The model under review builds one solid part; all positions refer to its coordinate system, in mm. A direction names the side the tool comes from. Round coordinates to 2 decimals unless told otherwise and drop trailing zeros. Loops run counter-clockwise (first coordinate to the right, second up) from the corner with the lowest first, then second, coordinate; pieces in that order, holes last. Notation, with made-up numbers: (77, 31.25) -> (136, 31.25) arc R18 cw to (136, 41.25) -> close; hole circle Ø3 at (73.25, 67). An arc over 180 degrees is marked (long way). Use a Markdown table: item, result. Add a question column.
1) Consider section D-D on y = 2.45. State how many separate pieces and enclosed holes the cut face has, plus the area to 3 significant figures.
2) For faces 1 (the flat face through (25, 1, 24)), 2 (the flat face through (9.833, 1, -23)), 3 (the flat face through (26.5, 1, 0)), list the 3-axis set-ups (+Z, -Z, +X, -X, +Y, -Y) from which the entire face can be reached by the end or side of a thin tool; tool diameter is ignored.
3) Wall thickness on probe 1 along X at (y, z) = (1.3, -15.69); probe 2 along Z at (x, y) = (-8, 0.5); probe 3 along X at (y, z) = (2.8, -22.5): over which ranges is each line inside the solid? List them lowest first.
4) Mouldability with a two-part tool opening along Z and no side actions: class faces 4 (the flat face through (29.5, 1, 16)), 5 (the flat face through (-26.5, 1, 0)), 6 (the flat face through (-28, 1, -8)), 7 (the flat face through (0, 2, -33)) as released by +Z, released by -Z, zero draft, split by the parting line, or undercut.
5) Insertion check: pin 1 (1.5 mm diameter, centred on x = -21, y = 0.5, fed in from -Z); pin 2 (0.9 mm diameter, centred on x = 26, y = 1, fed in from +Z); pin 3 (1.5 mm diameter, centred on y = 1.5, z = 1, fed in from +X). Each pin has a flat end and moves straight along its axis. Give the tip position at first contact, or say it passes through.
6) Consider section B-B on x = 0. Give the boundary of the cut face in (y, z).
7) Consider section C-C on z = -15.69. Give the boundary of the cut face in (x, y).
8) Consider section A-A on z = 28.5. Give the boundary of the cut face in (x, y).
from build123d import *

# Parameters (mm, degrees)
SKETCH1_R           = 1.6
BOSS_EXTRUDE1_DEPTH = 3
SKETCH2_R           = 2.1
BOSS_EXTRUDE2_DEPTH = 3


with BuildPart() as part:
    # Sketch1 → Boss-Extrude1 (new body)
    with BuildSketch(Plane(origin=(0, 0, 0), x_dir=(1, 0, 0), z_dir=(0, 1, 0))):
        Polygon((-29.5, 24), (-29.5, 8), (-26.5, 8), (-26.5, -8), (-29.5, -8), (-29.5, -24), (-9.833333333, -24), (-9.833333333, -21), (9.833333333, -21), (9.833333333, -24), (29.5, -24), (29.5, -8), (26.5, -8), (26.5, 8), (29.5, 8), (29.5, 24), (9.833333333, 24), (9.833333333, 21), (-9.833333333, 21), (-9.833333333, 24), align=None)
        with Locations(Location((-21.0185, 15.69, 0), (0, 0, 270))):
            Circle(SKETCH1_R, mode=Mode.SUBTRACT)
        with Locations(Location((21.0185, 15.69, 0), (0, 0, 270))):
            Circle(SKETCH1_R, mode=Mode.SUBTRACT)
        with Locations(Location((21.0185, -13.52, 0), (0, 0, 270))):
            Circle(SKETCH1_R, mode=Mode.SUBTRACT)
    extrude(amount=BOSS_EXTRUDE1_DEPTH)

    # Sketch2 → Boss-Extrude2 (add)
    with BuildSketch(Plane(origin=(0, 3, 0), x_dir=(1, 0, 0), z_dir=(0, 1, 0))):
        Polygon((-19.666666667, 24), (-9.833333333, 33), (9.833333333, 33), (19.666666667, 24), align=None)
        with Locations(Location((0, 28.5, 0), (0, 0, 270))):
            Circle(SKETCH2_R, mode=Mode.SUBTRACT)
    boss_extrude2 = extrude(amount=-BOSS_EXTRUDE2_DEPTH)

    # Mirror1: Boss-Extrude2 across plane
    add(boss_extrude2.mirror(Plane.XY))


solid = part.part
Result set:
| question | item | result |
|---|---|---|
| 1 | separate pieces | 1 |
| 1 | enclosed holes | 7 |
| 1 | area | 3,100 mm2 |
| 2 | face 1 | +Z, +X, +Y, -Y |
| 2 | face 2 | +Y, -Y |
| 2 | face 3 | +X, +Y, -Y |
| 3 | probe 1 | -29.5 to -22.62, -19.42 to 19.42, 22.62 to 29.5 |
| 3 | probe 2 | -33 to -24, -21 to 21, 24 to 33 |
| 3 | probe 3 | -29.5 to -9.83, 9.83 to 29.5 |
| 4 | face 4 | zero draft |
| 4 | face 5 | undercut |
| 4 | face 6 | undercut |
| 4 | face 7 | released by -Z |
| 5 | pin 1 | z = -24 |
| 5 | pin 2 | z = 24 |
| 5 | pin 3 | x = 26.5 |
| 6 | outline | (0, -33) -> (3, -33) -> (3, -30.6) -> (0, -30.6) -> close; (0, -26.4) -> (3, -26.4) -> (3, -24) -> (0, -24) -> close; (0, -21) -> (3, -21) -> (3, 21) -> (0, 21) -> close; (0, 24) -> (3, 24) -> (3, 26.4) -> (0, 26.4) -> close; (0, 30.6) -> (3, 30.6) -> (3, 33) -> (0, 33) -> close |
| 7 | outline | (-29.5, 0) -> (-22.62, 0) -> (-22.62, 3) -> (-29.5, 3) -> close; (-19.42, 0) -> (19.42, 0) -> (19.42, 3) -> (-19.42, 3) -> close; (22.62, 0) -> (29.5, 0) -> (29.5, 3) -> (22.62, 3) -> close |
| 8 | outline | (-14.75, 0) -> (-2.1, 0) -> (-2.1, 3) -> (-14.75, 3) -> close; (2.1, 0) -> (14.75, 0) -> (14.75, 3) -> (2.1, 3) -> close |
